Source: CAD feature listing. Evaluate the final solid. Frame: model axes, mm. A direction names the side the tool comes from. Round coordinates to 2 decimals unless told otherwise and drop trailing zeros. Order: outer loops, then holes, each group sorted by start corner. A loop starts at its lowest first (then second) coordinate and runs counter-clockwise, first axis right, second up. Notation, with made-up numbers: (40, -13) -> (88, -13) arc R19 ccw to (88, 19) -> close; hole circle Ø3 at (29, 74.5). An arc over 180 degrees is marked (long way). Use a Markdown table: item, result. Add a question column.
```python
from build123d import *

# Parameters (mm, degrees)
FILLET1_R          = 0.762
SKETCH3_R          = 13.90015
CUT_EXTRUDE1_DEPTH = 16.51


with BuildPart() as part:
    # Sketch2 → Revolve1 (revolve)
    with BuildSketch(Plane.XY, mode=Mode.PRIVATE) as revolve1_sk:
        with BuildLine():
            Line((6.35, -11.1125), (6.35, 11.1125))
            Line((6.35, 11.1125), (8.89, 11.1125))
            ThreePointArc((8.89, 11.1125), (9.690049959, 10.948371533), (10.360856835, 10.482500061))
            ThreePointArc((10.360856835, 10.482500061), (11.258914316, 9.934904036), (12.310452921, 9.909700708))
            Line((12.310452921, 9.909700708), (17.272, 11.1125))
            Line((17.272, 11.1125), (18.542, 11.1125))
            Line((18.542, 11.1125), (18.542, 10.6045))
            Line((18.542, 10.6045), (24.892, 10.6045))
            Line((24.892, 10.6045), (25.4, 0))
            Line((25.4, 0), (24.892, -10.6045))
            Line((24.892, -10.6045), (18.542, -10.6045))
            Line((18.542, -10.6045), (18.542, -11.1125))
            Line((18.542, -11.1125), (17.272, -11.1125))
            Line((17.272, -11.1125), (12.310452921, -9.909700708))
            ThreePointArc((12.310452921, -9.909700708), (11.258914316, -9.934904036), (10.360856835, -10.482500061))
            ThreePointArc((10.360856835, -10.482500061), (9.690049959, -10.948371533), (8.89, -11.1125))
            Line((8.89, -11.1125), (6.35, -11.1125))
        make_face()
    revolve(revolve1_sk.sketch.rotate(Axis((0, 0, 0), (0, 1, 0)), 90), axis=Axis((0, 0, 0), (0, 1, 0)))  # turned: the seam where the file's is

    # Fillet1
    fillet1_edges = [part.edges().sort_by_distance(p)[0] for p in [
        (0, -10.6045, 24.892),
        (0, 10.6045, 24.892),
    ]]
    fillet(fillet1_edges, radius=FILLET1_R)

    # Sketch3 → Cut-Extrude1 (cut)
    with BuildSketch(Plane(origin=(0, 11.1125, 0), x_dir=(-1, 0, 0), z_dir=(0, 1, 0))):
        with Locations(Location((0, 0, 0), (0, 0, 90))):  # turned: the seam where the file's is
            Circle(SKETCH3_R)
    extrude(amount=-CUT_EXTRUDE1_DEPTH, mode=Mode.SUBTRACT)


solid = part.part
```
1) Line query: probe 1 along X at (y, z) = (-0.25, 0); probe 2 along Y at (x, z) = (-18, 16); probe 3 along X at (y, z) = (2.25, -2). Output: solid intervals per line, ascending. Write a range as from..to.
2) Section A-A on y = 2. Output: boundary loops of the cut face in (x, z), then the cut area to 3 significant figures.
3) Reachability of faces 1 (the flat face through (14.2, -10.604, -12.4)), 2 (the flat face through (-6, -5.398, 3)), 3 (the flat face through (-17, -11.112, -5)) from +Z, -Z, +X, -X, +Y, -Y: full face, straight path, thin tool, end or side. Return the list, or none.
4) Draft query along X for faces 4 (the cylindrical face through (3.86, -8.21, 5.04)), 5 (the flat face through (-17, 11.112, 5)), 6 (the cylindrical face through (-12.53, -10.86, 13.67)). Return one class per face: pulls with the +X half, pulls with the -X half, needs draft (parallel to the pull), parting line crosses it, or undercut.
5) Section B-B on y = -7.75. Output: boundary loops of the cut face in (x, z), then the cut area to 3 significant figures.
6) First-contact query: pin 1 Ø2 at (x, z) = (-6, -14) entering from +Y; pin 2 Ø12 at (x, z) = (1, 9.5) entering from +Y; pin 3 Ø10 at (x, y) = (-6, -5) entering from -Z; pin 4 Ø5 at (x, z) = (-1, 1) entering from +Y. Flat tips, straight axial feed; report the tip coordinate or a pass-through.
Conclusion:
| question | item | result |
|---|---|---|
| 1 | probe 1 | x = -25.39..-13.9, 13.9..25.39 |
| 1 | probe 2 | y = -10.6..10.6 |
| 1 | probe 3 | x = -25.21..-13.76, 13.76..25.21 |
| 2 | outline | circle Ø50.61 at (0, 0); hole circle Ø27.8 at (0, 0) |
| 2 | area | 1,400 mm^2 |
| 3 | face 1 | -Y |
| 3 | face 2 | +Y |
| 3 | face 3 | +Z, -Z, +X, -X, -Y |
| 4 | face 4 | undercut |
| 4 | face 5 | needs draft |
| 4 | face 6 | parting line crosses it |
| 5 | outline | circle Ø50.06 at (0, 0); hole circle Ø12.7 at (0, 0) |
| 5 | area | 1,840 mm^2 |
| 6 | pin 1 | stops at y = 10.86 |
| 6 | pin 2 | stops at y = 10.7 |
| 6 | pin 3 | stops at z = -25.23 |
| 6 | pin 4 | passes through |
